Geometry check sheet. Reference: drawing and pictorial views, mm from the part's lowest x, y, z. Coordinates: 2 decimals unless noted, no trailing zeros. Write each loop counter-clockwise with the first axis right and the second up, starting at its lowest first coordinate (ties: lowest second). Pieces come first, ordered by that corner, then holes. Notation, with made-up numbers: M 1.5,-25.5 L 47.5,-25.5 A24 cw 47.5,6.5 Z; hole C 6,79 d6. An arc over 180 degrees is marked long. One line per item, written item: value.
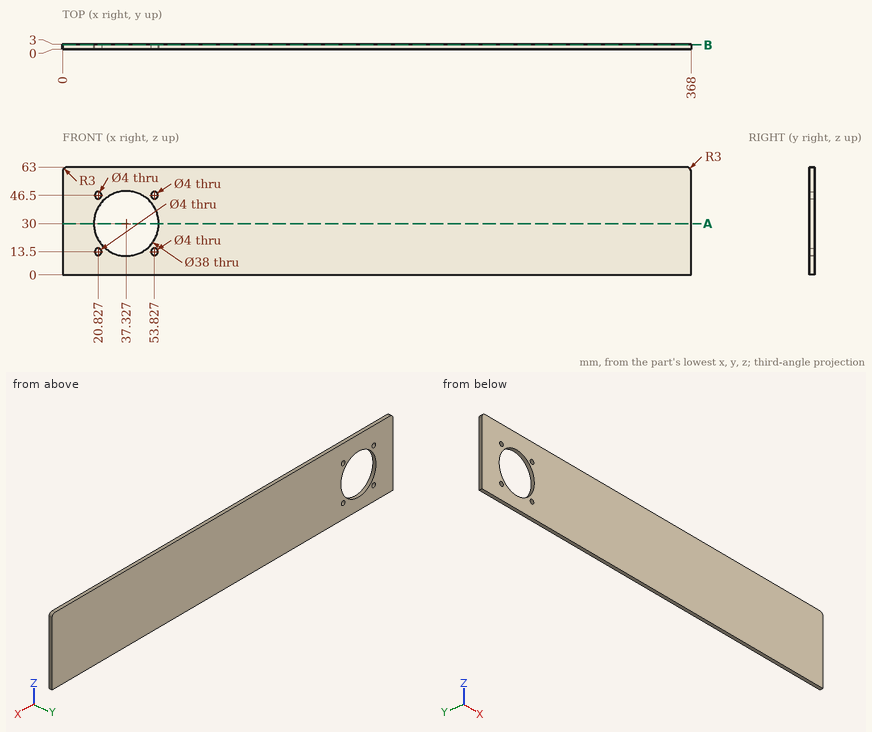
Item 1: Go/stop test with a flat-tipped pin: P1, Ø10, axis at x = 327, z = 46.5, coming from the -Y side. Record where the tip stops, or that it passes through.
The answers:
P1: stops at y = 0
Item 2: Cross-section at A-A, the plane z = 30. Enter the section's corners in (x, y), and give its area (3 significant figures).
The answers:
outline: M 0,0 L 18.33,0 L 18.33,3 L 0,3 Z; M 56.33,0 L 368,0 L 368,3 L 56.33,3 Z
area: 990 mm²
Item 3: Cross-section at B-B, the plane y = 2.5. Enter the section's corners in (x, z), and give its area (3 significant figures).
The answers:
outline: M 0,0 L 368,0 L 368,60 A3 ccw 365,63 L 3,63 A3 ccw 0,60 Z; hole C 37.33,30 d38; hole C 20.83,13.5 d4; hole C 20.83,46.5 d4; hole C 53.83,13.5 d4; hole C 53.83,46.5 d4
area: 22,000 mm²
Item 4: Scan lines: line 1 (X direction, y = 2.35, z = 30.5); line 2 (X direction, y = 1.95, z = 40). Record each from-to range of solid material in increasing order.
The answers:
line 1: x = 0 to 18.33, 56.32 to 368
line 2: x = 0 to 21.17, 53.48 to 368
